Read the model definition and answer for the solid it produces. Units are mm, in the model's axes. A direction names the side the tool comes from. Give positions to 0.01 mm unless a question says otherwise; leave off trailing zeros. Loops run counter-clockwise (first coordinate to the right, second up) from the corner with the lowest first, then second, coordinate; pieces in that order, holes last. Notation, with made-up numbers: (56, 20.25) - (105, 20.25) arc R23 cw to (105, 37.25) - close; hole circle Ø9 at (39, -5). An arc over 180 degrees is marked (long way). Write item = value, one per line.
```python
from build123d import *

# Parameters (mm, degrees)
SKETCH1_W           = 90
SKETCH1_H           = 70
SKETCH1_W_2         = 30
SKETCH1_R           = 2.025
SKETCH1_H_2         = 10
BOSS_EXTRUDE1_DEPTH = 2
SKETCH2_W           = 59
SKETCH2_H           = 90
BOSS_EXTRUDE2_DEPTH = 29
SKETCH4_W           = 55
SKETCH4_H           = 25
CUT_EXTRUDE1_DEPTH  = 87.5
FILLET1_R           = 1.5
FILLET2_R           = 0.4
FILLET3_R           = 10
FILLET7_R           = 2
SKETCH7_R           = 1.5
CUT_EXTRUDE2_DEPTH  = 5


with BuildPart() as part:
    # Sketch1 → Boss-Extrude1 (new body)
    # profile 1 of 5: a face of its own
    with BuildSketch(Plane(origin=(0, 0, 0), x_dir=(1, 0, 0), z_dir=(0, 1, 0))):
        Rectangle(SKETCH1_W, SKETCH1_H)
    # profile 2 of 5: a face of its own
    with BuildSketch(Plane(origin=(0, 0, 0), x_dir=(1, 0, 0), z_dir=(0, 1, 0))):
        with Locations((-60, 0)):
            Rectangle(SKETCH1_W_2, SKETCH1_H)
        with Locations(Location((-72, -25, 0), (0, 0, 270))):
            Circle(SKETCH1_R, mode=Mode.SUBTRACT)
        with Locations(Location((-72, 25, 0), (0, 0, 270))):
            Circle(SKETCH1_R, mode=Mode.SUBTRACT)
    # profile 3 of 5: a face of its own
    with BuildSketch(Plane(origin=(0, 0, 0), x_dir=(1, 0, 0), z_dir=(0, 1, 0))):
        with Locations((60, 0)):
            Rectangle(SKETCH1_W_2, SKETCH1_H)
        with Locations(Location((72, -25, 0), (0, 0, 270))):
            Circle(SKETCH1_R, mode=Mode.SUBTRACT)
        with Locations(Location((72, 25, 0), (0, 0, 270))):
            Circle(SKETCH1_R, mode=Mode.SUBTRACT)
    # profile 4 of 5: a face of its own
    with BuildSketch(Plane(origin=(0, 0, 0), x_dir=(1, 0, 0), z_dir=(0, 1, 0))):
        with Locations((0, -40)):
            Rectangle(SKETCH1_W, SKETCH1_H_2)
    # profile 5 of 5: a face of its own
    with BuildSketch(Plane(origin=(0, 0, 0), x_dir=(1, 0, 0), z_dir=(0, 1, 0))):
        with Locations((0, 40)):
            Rectangle(SKETCH1_W, SKETCH1_H_2)
    extrude(amount=BOSS_EXTRUDE1_DEPTH)

    # Sketch2 → Boss-Extrude2 (add)
    with BuildSketch(Plane(origin=(0, 2, 0), x_dir=(1, 0, 0), z_dir=(0, 1, 0))):
        Rectangle(SKETCH2_W, SKETCH2_H)
    extrude(amount=BOSS_EXTRUDE2_DEPTH)

    # Sketch4 → Cut-Extrude1 (cut)
    with BuildSketch(Plane.XY.offset(45)):
        with Locations((0, 16.5)):
            Rectangle(SKETCH4_W, SKETCH4_H)
    extrude(amount=-CUT_EXTRUDE1_DEPTH, mode=Mode.SUBTRACT)

    # Fillet1
    fillet1_edges = [part.edges().sort_by_distance(p)[0] for p in [
        (-29.5, 2, 0),
        (29.5, 2, 0),
        (-29.5, 31, 0),
        (29.5, 31, 0),
    ]]
    fillet(fillet1_edges, radius=FILLET1_R)

    # Fillet2
    fillet2_edges = [part.edges().sort_by_distance(p)[0] for p in [
        (-27.5, 4, 1.25),
        (0, 29, -42.5),
        (-27.5, 29, 1.25),
        (27.5, 16.5, -42.5),
        (27.5, 29, 1.25),
        (27.5, 4, 1.25),
        (-27.5, 16.5, -42.5),
        (0, 4, -42.5),
    ]]
    fillet(fillet2_edges, radius=FILLET2_R)

    # Fillet3
    fillet3_edges = [part.edges().sort_by_distance(p)[0] for p in [
        (-45, 1, 35),
        (-45, 1, -35),
        (45, 1, -35),
        (45, 1, 35),
    ]]
    fillet(fillet3_edges, radius=FILLET3_R - 0.0001)  # a hair under: the kernel refuses the full size

    # Fillet7
    fillet7_edges = [part.edges().sort_by_distance(p)[0] for p in [
        (-45, 1, -45),
        (45, 1, -45),
        (75, 1, -35),
        (75, 1, 35),
        (45, 1, 45),
        (-45, 1, 45),
        (-75, 1, 35),
        (-75, 1, -35),
    ]]
    fillet(fillet7_edges, radius=FILLET7_R)

    # Sketch7 → Cut-Extrude2 (cut)
    with BuildSketch(Plane(origin=(0, 31, 0), x_dir=(1, 0, 0), z_dir=(0, 1, 0))):
        with Locations(Location((-12.5, 33.5, 0), (0, 0, 270))):
            Circle(SKETCH7_R)
        with Locations(Location((22.5, 33.5, 0), (0, 0, 270))):
            Circle(SKETCH7_R)
        with Locations(Location((22.5, -11.5, 0), (0, 0, 270))):
            Circle(SKETCH7_R)
        with Locations(Location((-12.5, -11.5, 0), (0, 0, 270))):
            Circle(SKETCH7_R)
    extrude(amount=-CUT_EXTRUDE2_DEPTH, mode=Mode.SUBTRACT)


solid = part.part
```
1) A cutting plane is placed at D-D on z = 17. Determine the outline of the cut face in (x, y), then the cut area to 3 significant figures.
Output:
outline = (-75, 0) - (75, 0) - (75, 2) - (31, 2) arc R1.5 cw to (29.5, 3.5) - (29.5, 29.5) arc R1.5 ccw to (28, 31) - (-28, 31) arc R1.5 ccw to (-29.5, 29.5) - (-29.5, 3.5) arc R1.5 cw to (-31, 2) - (-75, 2) - close; hole (-27.5, 4.4) arc R0.4 ccw to (-27.1, 4) - (27.1, 4) arc R0.4 ccw to (27.5, 4.4) - (27.5, 28.6) arc R0.4 ccw to (27.1, 29) - (-27.1, 29) arc R0.4 ccw to (-27.5, 28.6) - close
area = 636 mm²
2) A cutting plane is placed at A-A on z = -25. Determine the outline of the cut face in (x, y) (3 decimals), then the cut area to 3 significant figures.
Output:
outline = (-75, 0) - (-74.025, 0) - (-74.025, 2) - (-75, 2) - close; (-69.975, 0) - (69.975, 0) - (69.975, 2) - (31, 2) arc R1.5 cw to (29.5, 3.5) - (29.5, 29.5) arc R1.5 ccw to (28, 31) - (-28, 31) arc R1.5 ccw to (-29.5, 29.5) - (-29.5, 3.5) arc R1.5 cw to (-31, 2) - (-69.975, 2) - close; (74.025, 0) - (75, 0) - (75, 2) - (74.025, 2) - close; hole (-27.5, 4.4) arc R0.4 ccw to (-27.1, 4) - (27.1, 4) arc R0.4 ccw to (27.5, 4.4) - (27.5, 28.6) arc R0.4 ccw to (27.1, 29) - (-27.1, 29) arc R0.4 ccw to (-27.5, 28.6) - close
area = 620 mm²
3) A tool of negligible diameter and unlimited length cuts with its end or side. For faces 4 (the face through (73.37, 0.99, 23.51)), 5 (the face through (27.5, 16, 2)), 6 (the face through (-29.5, 16, 1)), 7 (the face through (29.5, 16, 1)), 8 (the face through (-12.43, 30.01, 10)), from which of +Z, -Z, +X, -X, +Y, -Y can it reach the whole face along a straight path? Write none if from no direction.
Output:
face_4 = +Y, -Y
face_5 = +Z
face_6 = +Z, -Z, -X, +Y
face_7 = +Z, -Z, +X, +Y
face_8 = +Y
4) A cutting plane is placed at C-C on y = 17.5. Determine the outline of the cut face in (x, z), then the cut area to 3 significant figures.
Output:
outline = (-29.5, -45) - (29.5, -45) - (29.5, 45) - (27.5, 45) - (27.5, -42.1) arc R0.4 cw to (27.1, -42.5) - (-27.1, -42.5) arc R0.4 cw to (-27.5, -42.1) - (-27.5, 45) - (-29.5, 45) - close
area = 498 mm²
5) A cutting plane is placed at B-B on x = 22.5. Determine the outline of the cut face in (y, z).
Output:
outline = (0, -45) - (31, -45) - (31, -35) - (29, -35) - (29, -42.1) arc R0.4 cw to (28.6, -42.5) - (4.4, -42.5) arc R0.4 cw to (4, -42.1) - (4, 45) - (0, 45) - close; (29, -32) - (31, -32) - (31, 10) - (29, 10) - close; (29, 13) - (31, 13) - (31, 45) - (29, 45) - close
6) Each of these flat-tipped pins is pushed along its axis until it touches: P1, Ø0.6, axis at x = 67.5, y = 0.5, coming from the +Z side; P2, Ø5, axis at y = 19.5, z = -34, coming from the -X side; P3, Ø2.5, axis at x = 22.5, z = -33.5, coming from the +Y side. Where does it stop, or does it pass through?
Output:
P1 = 35
P2 = -29.5
P3 = 4
7) Find the intervals of material crossed by probe 1 along X at (y, z) = (0.55, -25) (3 decimals); probe 2 along Y at (x, z) = (5.5, 14.5); probe 3 along X at (y, z) = (27, -9), in increasing order.
Output:
probe_1 = -75 to -74.025, -69.975 to 69.975, 74.025 to 75
probe_2 = 0 to 4, 29 to 31
probe_3 = -29.5 to -27.5, 27.5 to 29.5
8) The mould has two halves that part along Y. Classify faces 1 (the face through (-27.5, 16, 2)), 2 (the face through (-1, 15, -45)), 3 (the face through (-1, 0, -1)): pulls with the +Y half, pulls with the -Y half, needs draft (parallel to the pull), parting line crosses it, or undercut.
Output:
face_1 = undercut
face_2 = needs draft
face_3 = pulls with the -Y half
